from build123d import *

# Parameters (mm, degrees)
BOSS_EXTRUDE1_DEPTH = 25.4
SKETCH2_R           = 3.175
CUT_EXTRUDE2_DEPTH  = 20.05
SKETCH4_R           = 1.8288
CUT_EXTRUDE3_DEPTH  = 7.096


with BuildPart() as part:
    # Sketch1 → Boss-Extrude1 (new body)
    with BuildSketch(Plane(origin=(0, 0, 0), x_dir=(0, 0, -1), z_dir=(1, 0, 0))):
        Polygon((0, 6.096), (0, 0), (6.35, 0), (6.35, 2.921), (12.7, 2.921), (12.7, 0), (19.05, 0), (19.05, 6.096), align=None)
    extrude(amount=BOSS_EXTRUDE1_DEPTH)

    # Sketch2 → Cut-Extrude2 (cut, through all)
    with BuildSketch(Plane.XY):
        with Locations((12.7, -0.254)):
            Circle(SKETCH2_R)
    extrude(amount=-CUT_EXTRUDE2_DEPTH, mode=Mode.SUBTRACT)

    # Sketch4 → Cut-Extrude3 (cut, through all)
    with BuildSketch(Plane.XZ):
        with Locations((3.175, -3.175)):
            Circle(SKETCH4_R)
        with Locations((3.175, -15.875)):
            Circle(SKETCH4_R)
        with Locations((22.225, -3.175)):
            Circle(SKETCH4_R)
        with Locations((22.225, -15.875)):
            Circle(SKETCH4_R)
    extrude(amount=-CUT_EXTRUDE3_DEPTH, mode=Mode.SUBTRACT)


solid = part.part
Work out the finished part from the listing and answer in its coordinate system (mm). A direction names the side the tool comes from. Give positions to 0.01 mm unless a question says otherwise; leave off trailing zeros. Loops run counter-clockwise (first coordinate to the right, second up) from the corner with the lowest first, then second, coordinate; pieces in that order, holes last. Notation, with made-up numbers: (70.25, -40) - (78.25, -40) arc R25 cw to (78.25, -5) - close; hole circle Ø6 at (-6, 55.25). An arc over 180 degrees is marked (long way). Answer in a Markdown table with one row per item. Add a question column.
Q1. The part is cut by section D-D (x = 20.75). Determine the outline of the cut face in (y, z), and give its area (3 significant figures).
Q2. The part is cut by section B-B (z = -15.5). Determine the outline of the cut face in (x, y) (3 decimals), and give its area (3 significant figures).
Q3. The part is cut by section C-C (x = 17). Determine the outline of the cut face in (y, z).
Q4. The part is cut by section A-A (y = 1.75). Determine the outline of the cut face in (x, z) (3 decimals), and give its area (3 significant figures).
Q5. A tool of negligible diameter and unlimited length cuts with its end or side. For faces 4 (the flat face through (20, 0, -16)), 5 (the flat face through (20, 1, -12.7)), from which of +Z, -Z, +X, -X, +Y, -Y can it reach the whole face along a straight path? Write none if from no direction.
Q6. Determine the mould class of faces 1 (the cylindrical face through (12.77, 2.92, -3.13)), 2 (the flat face through (25.4, 3.1, -9.4)), 3 (the flat face through (5, 1, -12.7)) for opening direction X: released by +X, released by -X, zero draft, split by the parting line, or undercut.
Q7. Each of these flat-tipped pins is pushed along its axis until it touches: P1, Ø3.5, axis at x = 3.175, z = -15.875, coming from the +Y side; P2, Ø1.9, axis at x = 17.5, z = -9, coming from the -Y side. Where does it stop, or does it pass through?
Q8. Consider line 1 along X through (y, z) = (1, -2.75); line 2 along X through (y, z) = (2.5, -15); line 3 along Z through (x, y) = (20.75, 5). Determine where each line is inside the solid, lowest interval first.
Solution:
| question | item | result |
|---|---|---|
| 1 | outline | (0, -19.05) - (6.1, -19.05) - (6.1, -16.96) - (0, -16.96) - close; (0, -14.79) - (6.1, -14.79) - (6.1, -4.26) - (0, -4.26) - (0, -6.35) - (2.92, -6.35) - (2.92, -12.7) - (0, -12.7) - close; (0, -2.09) - (6.1, -2.09) - (6.1, 0) - (0, 0) - close |
| 1 | area | 71.2 mm² |
| 2 | outline | (0, 0) - (1.385, 0) - (1.385, 6.096) - (0, 6.096) - close; (4.965, 0) - (9.535, 0) arc R3.175 cw to (15.865, 0) - (20.435, 0) - (20.435, 6.096) - (4.965, 6.096) - close; (24.015, 0) - (25.4, 0) - (25.4, 6.096) - (24.015, 6.096) - close |
| 2 | area | 97.0 mm² |
| 3 | outline | (0, -19.05) - (6.1, -19.05) - (6.1, 0) - (0, 0) - (0, -6.35) - (2.92, -6.35) - (2.92, -12.7) - (0, -12.7) - close |
| 4 | outline | (0, -19.05) - (10.237, -19.05) - (10.237, -12.7) - (0, -12.7) - close; (0, -6.35) - (10.237, -6.35) - (10.237, 0) - (0, 0) - close; (15.163, -19.05) - (25.4, -19.05) - (25.4, -12.7) - (15.163, -12.7) - close; (15.163, -6.35) - (25.4, -6.35) - (25.4, 0) - (15.163, 0) - close; hole circle Ø3.658 at (3.175, -15.875); hole circle Ø3.658 at (3.175, -3.175); hole circle Ø3.658 at (22.225, -15.875); hole circle Ø3.658 at (22.225, -3.175) |
| 4 | area | 218 mm² |
| 5 | face 4 | +Z, -Z, +X, -X, -Y |
| 5 | face 5 | +X, -X, -Y |
| 6 | face 1 | undercut |
| 6 | face 2 | released by +X |
| 6 | face 3 | zero draft |
| 7 | P1 | passes through |
| 7 | P2 | stops at y = 2.92 |
| 8 | line 1 | x = 0 to 1.4, 4.95 to 9.78, 15.62 to 20.45, 24 to 25.4 |
| 8 | line 2 | x = 0 to 1.57, 4.78 to 11.12, 14.28 to 20.62, 23.83 to 25.4 |
| 8 | line 3 | z = -19.05 to -16.96, -14.79 to -4.26, -2.09 to 0 |
